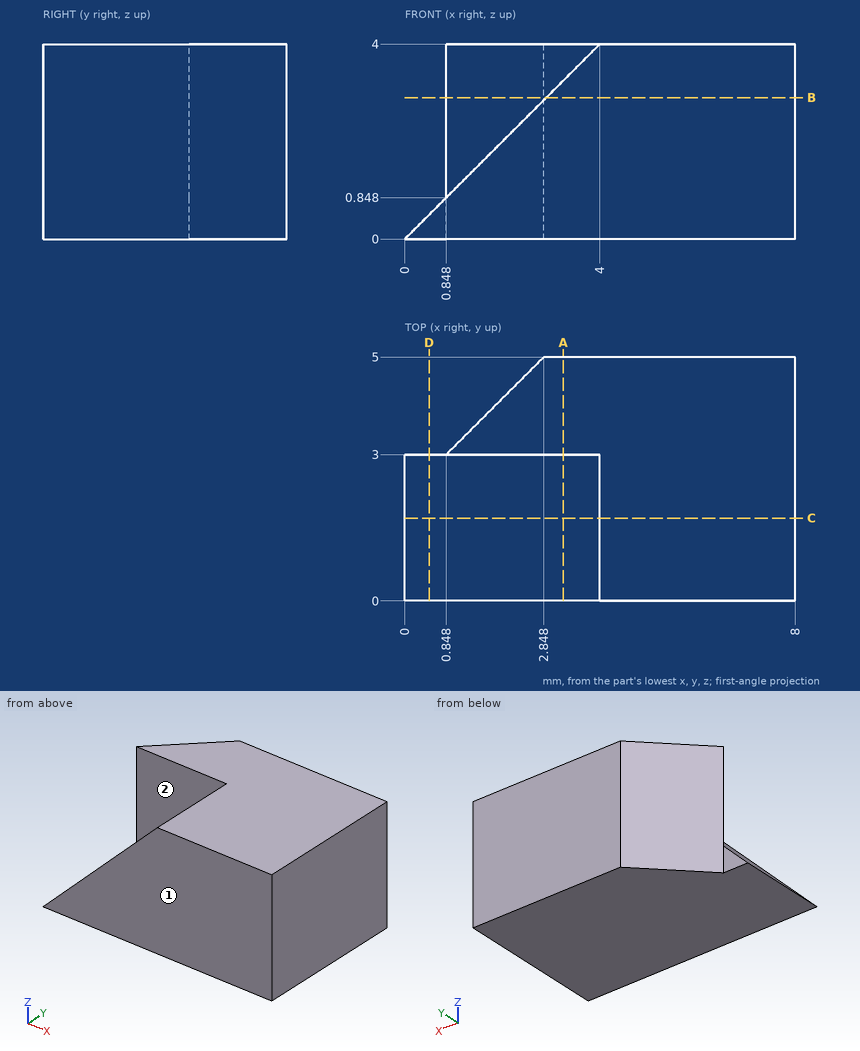
The figure shows three views and two pictorial views of one solid part (mm, origin at its lowest corner). Answer the questions. A direction names the side the tool comes from. Give positions to 0.01 mm unless a question says otherwise; leave off trailing zeros. Write each loop counter-clockwise with the first axis right and the second up, starting at its lowest first coordinate (ties: lowest second). Pieces come first, ordered by that corner, then holes. Notation, with made-up numbers: (-13.5, -6) - (22.5, -6) arc R9 ccw to (22.5, 4) - close; hole circle Ø2 at (41, -32.5). An arc over 180 degrees is marked (long way). Use one line per item in the form item = value. Start each with the question number.
1) Consider line 1 along X through (y, z) = (1.25, 1.6); line 2 along Y through (x, z) = (1, 0.35); line 3 along Z through (x, y) = (1.75, 1.1). Determine where each line is inside the solid, lowest interval first. Write a range as from..to.
2) Find section A-A on x = 3.25. Determine the outline of the cut face in (y, z).
3) Find section B-B on z = 2.9. Determine the outline of the cut face in (x, y), plus the area to 3 significant figures.
4) A tool of negligible diameter and unlimited length cuts with its end or side. For the marked faces 1 and 2, from which of +Z, -Z, +X, -X, +Y, -Y can it reach the whole face along a straight path? Write none if from no direction.
5) Find section D-D on x = 0.5. Determine the outline of the cut face in (y, z), plus the area to 3 significant figures.
6) Find section C-C on y = 1.7. Determine the outline of the cut face in (x, z), plus the area to 3 significant figures.
Geometry results:
q1.line_1 = 1.6..8
q1.line_2 = 0..3.15
q1.line_3 = 0..1.75
q2.outline = (0, 0) - (5, 0) - (5, 4) - (3, 4) - (3, 3.25) - (0, 3.25) - close
q3.outline = (0.85, 3) - (2.9, 3) - (2.9, 0) - (8, 0) - (8, 5) - (2.85, 5) - close
q3.area = 27.6 mm2
q4.face_1 = +Z, -Z, +X, -X, -Y
q4.face_2 = +Z, -X, -Y
q5.outline = (0, 0) - (3, 0) - (3, 0.5) - (0, 0.5) - close
q5.area = 1.50 mm2
q6.outline = (0, 0) - (8, 0) - (8, 4) - (4, 4) - close
q6.area = 24.0 mm2
